Geometry check sheet. Reference: the model listing, model coordinates, mm. Face numbers are marked on the shaded views. A direction names the side the tool comes from. Round coordinates to 2 decimals unless told otherwise and drop trailing zeros. Write each loop counter-clockwise with the first axis right and the second up, starting at its lowest first coordinate (ties: lowest second). Pieces come first, ordered by that corner, then holes. Notation, with made-up numbers: (35.5, -13.5) -> (62.5, -13.5) arc R26 cw to (62.5, 16.5) -> close; hole circle Ø2 at (76.25, -8). An arc over 180 degrees is marked (long way). Return JSON: item names as keys, results as strings. Group by question number.
from build123d import *

# Parameters (mm, degrees)
SKETCH1_R                       = 2.5
BOSS_EXTRUDE1_DEPTH             = 27
SKETCH2_R                       = 11
BOSS_EXTRUDE2_DEPTH             = 2
SKETCH3_W                       = 42.418
SKETCH3_H                       = 42.418
BOSS_EXTRUDE3_DEPTH             = 48
CUT_EXTRUDE1_DEPTH              = 76
M3X0_5_TAPPED_HOLE1_D           = 2.5
M3X0_5_TAPPED_HOLE1_DEPTH       = 7.5
M3X0_5_TAPPED_HOLE1_CBORE_D     = 3
M3X0_5_TAPPED_HOLE1_CBORE_DEPTH = 6
M3X0_5_TAPPED_HOLE1_TIP         = 0.751075774
CUT_EXTRUDE3_DEPTH              = 15.25
CUT_EXTRUDE3_DEPTH_BACK         = 15.25
SKETCH9_W                       = 16
SKETCH9_H                       = 4.5
BOSS_EXTRUDE4_DEPTH             = 4.75


with BuildPart() as part:
    # Sketch1 → Boss-Extrude1 (new body)
    with BuildSketch(Plane.XY):
        Circle(SKETCH1_R)
    extrude(amount=BOSS_EXTRUDE1_DEPTH)

    # Sketch2 → Boss-Extrude2 (add)
    with BuildSketch(Plane(origin=(0, 0, 0), x_dir=(-1, 0, 0), z_dir=(0, 0, -1))):
        Circle(SKETCH2_R)
    extrude(amount=-BOSS_EXTRUDE2_DEPTH)

    # Sketch3 → Boss-Extrude3 (add)
    with BuildSketch(Plane(origin=(0, 0, 0), x_dir=(-1, 0, 0), z_dir=(0, 0, -1))):
        Rectangle(SKETCH3_W, SKETCH3_H)
    extrude(amount=BOSS_EXTRUDE3_DEPTH)

    # Sketch4 → Cut-Extrude1 (cut, through all)
    with BuildSketch(Plane(origin=(0, 0, -48), x_dir=(-1, 0, 0), z_dir=(0, 0, -1))):
        with BuildLine():
            Line((-21.209, -15.887992919), (-21.209, -21.209))
            Line((-21.209, -21.209), (-15.887992919, -21.209))
            ThreePointArc((-15.887992919, -21.209), (-18.738329701, -18.738329701), (-21.209, -15.887992919))
        make_face()
        with BuildLine():
            Line((15.887992919, -21.209), (21.209, -21.209))
            Line((21.209, -21.209), (21.209, -15.887992919))
            ThreePointArc((21.209, -15.887992919), (18.738329701, -18.738329701), (15.887992919, -21.209))
        make_face()
        with BuildLine():
            Line((21.209, 15.887992919), (21.209, 21.209))
            Line((21.209, 21.209), (15.887992919, 21.209))
            ThreePointArc((15.887992919, 21.209), (18.738329701, 18.738329701), (21.209, 15.887992919))
        make_face()
        with BuildLine():
            Line((-15.887992919, 21.209), (-21.209, 21.209))
            Line((-21.209, 21.209), (-21.209, 15.887992919))
            ThreePointArc((-21.209, 15.887992919), (-18.738329701, 18.738329701), (-15.887992919, 21.209))
        make_face()
    extrude(amount=-CUT_EXTRUDE1_DEPTH, mode=Mode.SUBTRACT)

    # M3x0.5 Tapped Hole1
    with Locations(Plane.XY):
        with Locations((-15.5, 15.5), (-15.5, -15.5), (15.5, -15.5), (15.5, 15.5)):
            CounterBoreHole(M3X0_5_TAPPED_HOLE1_D / 2, M3X0_5_TAPPED_HOLE1_CBORE_D / 2, M3X0_5_TAPPED_HOLE1_CBORE_DEPTH, depth=M3X0_5_TAPPED_HOLE1_DEPTH)
            with Locations((0, 0, -(M3X0_5_TAPPED_HOLE1_DEPTH + M3X0_5_TAPPED_HOLE1_TIP / 2))):  # 118° drill point
                Cone(0, M3X0_5_TAPPED_HOLE1_D / 2, M3X0_5_TAPPED_HOLE1_TIP, mode=Mode.SUBTRACT)

    # Sketch8 → Cut-Extrude3 (cut, two sides)
    with BuildSketch(Plane.XY.offset(-24)) as cut_extrude3_sk:
        with BuildLine():
            Line((15.887992919, 21.209), (-15.887992919, 21.209))
            ThreePointArc((-15.887992919, 21.209), (-18.738329701, 18.738329701), (-21.209, 15.887992919))
            Line((-21.209, 15.887992919), (-21.209, -15.887992919))
            ThreePointArc((-21.209, -15.887992919), (-18.738329701, -18.738329701), (-15.887992919, -21.209))
            Line((-15.887992919, -21.209), (15.887992919, -21.209))
            ThreePointArc((15.887992919, -21.209), (18.738329701, -18.738329701), (21.209, -15.887992919))
            Line((21.209, -15.887992919), (21.209, 15.887992919))
            ThreePointArc((21.209, 15.887992919), (18.738329701, 18.738329701), (15.887992919, 21.209))
        make_face()
        with BuildLine():
            Line((-13.394406258, 21.109), (13.394406258, 21.109))
            ThreePointArc((13.394406258, 21.109), (17.67766953, 17.67766953), (21.109, 13.394406258))
            Line((21.109, 13.394406258), (21.109, -13.394406258))
            ThreePointArc((21.109, -13.394406258), (17.67766953, -17.67766953), (13.394406258, -21.109))
            Line((13.394406258, -21.109), (-13.394406258, -21.109))
            ThreePointArc((-13.394406258, -21.109), (-17.67766953, -17.67766953), (-21.109, -13.394406258))
            Line((-21.109, -13.394406258), (-21.109, 13.394406258))
            ThreePointArc((-21.109, 13.394406258), (-17.67766953, 17.67766953), (-13.394406258, 21.109))
        make_face(mode=Mode.SUBTRACT)
    extrude(amount=CUT_EXTRUDE3_DEPTH, mode=Mode.SUBTRACT)
    extrude(cut_extrude3_sk.sketch, amount=-CUT_EXTRUDE3_DEPTH_BACK, mode=Mode.SUBTRACT)

    # Sketch9 → Boss-Extrude4 (add)
    with BuildSketch(Plane.XZ.offset(21.209)):
        with Locations((0, -45.75)):
            Rectangle(SKETCH9_W, SKETCH9_H)
    extrude(amount=BOSS_EXTRUDE4_DEPTH)


solid = part.part
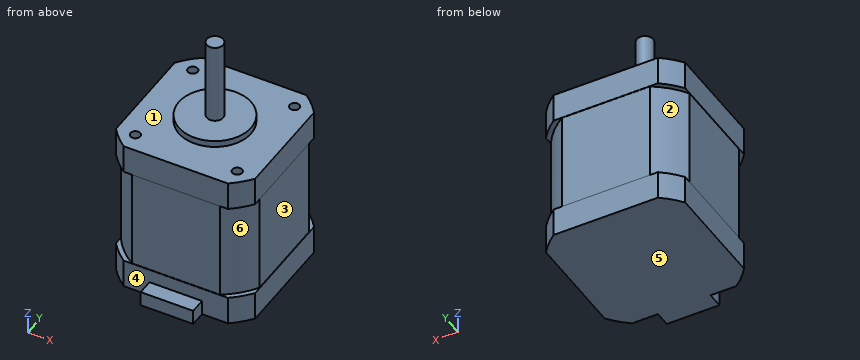
1) Go/stop test with flat-tipped pins: P1, Ø6, axis at x = 13.5, y = -9, coming from the +Z side; P2, Ø2, axis at x = 15.5, y = -15.5, coming from the +Z side; P3, Ø10, axis at y = -9, z = -22.5, coming from the +X side. Record where each tip stops, or that it passes through.
2) Mould release check, pull along Z, two halves, no side actions. Record for the marked faces 4, 5 and 6: +Z half, -Z half, draft (parallel to the pull), parting line (faces both ways), or undercut.
3) Sectioned sample at C-C on z = -19.5. Enter the section's corners in (x, y), and give its area (3 significant figures).
4) Sectioned sample at D-D on x = 18. Enter the section's corners in (y, z).
5) Sectioned sample at B-B on y = 0. Enter the section's corners in (x, z), and give its area (3 significant figures).
6) Sectioned sample at A-A on x = 0. Enter the section's corners in (y, z).
7) Tool access check on the marked faces 1, 2 and 3. Record the directions out of +Z, -Z, +X, -X, +Y, -Y that give a thin tool (end or side, any length) a straight path to the whole face; none if there is none.
8) Material ranges on probe 1 along Y at (x, z) = (15.5, -2.1); probe 2 along X at (y, z) = (15.5, -6.9); probe 3 along Z at (x, y) = (-19, 1), recorded low to high. Write a range as [from, to].
Evaluation:
{
 "1": {"P1": "stops at z = 0", "P2": "stops at z = -7.65", "P3": "stops at x = 21.11"},
 "2": {"face 4": "draft", "face 5": "-Z half", "face 6": "undercut"},
 "3": {"outline": "(-21.11, -13.39) arc R25 ccw to (-13.39, -21.11) -> (13.39, -21.11) arc R25 ccw to (21.11, -13.39) -> (21.11, 13.39) arc R25 ccw to (13.39, 21.11) -> (-13.39, 21.11) arc R25 ccw to (-21.11, 13.39) -> close", "area": "1,680 mm2"},
 "4": {"outline": "(-19.45, -48) -> (19.45, -48) -> (19.45, -39.25) -> (17.35, -39.25) -> (17.35, -8.75) -> (19.45, -8.75) -> (19.45, 0) -> (-19.45, 0) -> (-19.45, -8.75) -> (-17.35, -8.75) -> (-17.35, -39.25) -> (-19.45, -39.25) -> close"},
 "5": {"outline": "(-21.21, -48) -> (21.21, -48) -> (21.21, -39.25) -> (21.11, -39.25) -> (21.11, -8.75) -> (21.21, -8.75) -> (21.21, 0) -> (11, 0) -> (11, 2) -> (2.5, 2) -> (2.5, 27) -> (-2.5, 27) -> (-2.5, 2) -> (-11, 2) -> (-11, 0) -> (-21.21, 0) -> (-21.21, -8.75) -> (-21.11, -8.75) -> (-21.11, -39.25) -> (-21.21, -39.25) -> close", "area": "2,200 mm2"},
 "6": {"outline": "(-25.96, -48) -> (21.21, -48) -> (21.21, -39.25) -> (21.11, -39.25) -> (21.11, -8.75) -> (21.21, -8.75) -> (21.21, 0) -> (11, 0) -> (11, 2) -> (2.5, 2) -> (2.5, 27) -> (-2.5, 27) -> (-2.5, 2) -> (-11, 2) -> (-11, 0) -> (-21.21, 0) -> (-21.21, -8.75) -> (-21.11, -8.75) -> (-21.11, -39.25) -> (-21.21, -39.25) -> (-21.21, -43.5) -> (-25.96, -43.5) -> close"},
 "7": {"face 1": "+Z", "face 2": "-X, +Y", "face 3": "+X, +Y, -Y"},
 "8": {"probe 1": "y = [-21.21, -17], [-14, 14], [17, 21.21]", "probe 2": "x = [-21.21, -16.75], [-14.25, 14.25], [16.75, 21.21]", "probe 3": "z = [-48, 0]"}
}
